```python
from build123d import *

# Parameters (mm, degrees)
F0_R     = 12
F1_DEPTH = 3


with BuildPart() as f1:
    # F0 (on Top) → F1 (new body)
    with BuildSketch(Plane.XY):
        with BuildLine():
            Line((5, 16.248077), (5, 122.001923))
            ThreePointArc((5, 122.001923), (0, 155.25), (-5, 122.001923))
            Line((-5, 122.001923), (-5, 16.248077))
            ThreePointArc((-5, 16.248077), (-8.5, 14.722432), (-11.571247, 12.454165))
            Line((-11.571247, 12.454165), (-103.156765, 65.331089))
            ThreePointArc((-103.156765, 65.331089), (-134.450444, 77.625), (-108.156765, 56.670835))
            Line((-108.156765, 56.670835), (-16.571247, 3.793911))
            ThreePointArc((-16.571247, 3.793911), (-17, 0), (-16.571247, -3.793911))
            Line((-16.571247, -3.793911), (-108.156765, -56.670835))
            ThreePointArc((-108.156765, -56.670835), (-134.450444, -77.625), (-103.156765, -65.331089))
            Line((-103.156765, -65.331089), (-11.571247, -12.454165))
            ThreePointArc((-11.571247, -12.454165), (-8.5, -14.722432), (-5, -16.248077))
            Line((-5, -16.248077), (-5, -122.001923))
            ThreePointArc((-5, -122.001923), (0, -155.25), (5, -122.001923))
            Line((5, -122.001923), (5, -16.248077))
            ThreePointArc((5, -16.248077), (8.5, -14.722432), (11.571247, -12.454165))
            Line((11.571247, -12.454165), (103.156765, -65.331089))
            ThreePointArc((103.156765, -65.331089), (134.450444, -77.625), (108.156765, -56.670835))
            Line((108.156765, -56.670835), (16.571247, -3.793911))
            ThreePointArc((16.571247, -3.793911), (17, 0), (16.571247, 3.793911))
            Line((16.571247, 3.793911), (108.156765, 56.670835))
            ThreePointArc((108.156765, 56.670835), (134.450444, 77.625), (103.156765, 65.331089))
            Line((103.156765, 65.331089), (11.571247, 12.454165))
            ThreePointArc((11.571247, 12.454165), (8.5, 14.722432), (5, 16.248077))
        make_face()
        with Locations((-119.728012, -69.125)):
            Circle(F0_R, mode=Mode.SUBTRACT)
        with Locations((0, -138.25)):
            Circle(F0_R, mode=Mode.SUBTRACT)
        with Locations((119.728012, -69.125)):
            Circle(F0_R, mode=Mode.SUBTRACT)
        with Locations((-119.728012, 69.125)):
            Circle(F0_R, mode=Mode.SUBTRACT)
        Circle(F0_R, mode=Mode.SUBTRACT)
        with Locations((119.728012, 69.125)):
            Circle(F0_R, mode=Mode.SUBTRACT)
        with Locations((0, 138.25)):
            Circle(F0_R, mode=Mode.SUBTRACT)
    extrude(amount=F1_DEPTH)


solid = f1.part
```
Input: part model. Units: mm. Frame: model coordinates. Coordinates: 2 decimals unless noted, no trailing zeros. Loops run counter-clockwise (first coordinate to the right, second up) from the corner with the lowest first, then second, coordinate; pieces in that order, holes last.
Q1. Section D-D, the plane y = -44. Return the cut outline in (x, z).
Results are:
outline: (-86.21, 0) - (-66.21, 0) - (-66.21, 3) - (-86.21, 3) - close; (-5, 0) - (5, 0) - (5, 3) - (-5, 3) - close; (66.21, 0) - (86.21, 0) - (86.21, 3) - (66.21, 3) - close
Q2. Section B-B, the plane x = 0. Return the cut outline in (y, z), and give its area (4 significant figures).
Results are:
outline: (-155.25, 0) - (-150.25, 0) - (-150.25, 3) - (-155.25, 3) - close; (-126.25, 0) - (-12, 0) - (-12, 3) - (-126.25, 3) - close; (12, 0) - (126.25, 0) - (126.25, 3) - (12, 3) - close; (150.25, 0) - (155.25, 0) - (155.25, 3) - (150.25, 3) - close
area: 715.5 mm2
Q3. Mould query, pull axis Y, two halves, no side actions, for faces 1 (the cylindrical face through (134.101, -78.204, 1.479)), 2 (the flat face through (-0.6, 12.2, 0)), 3 (the flat face through (61.72, 29.86, 1.48)). Classes: +Y half, -Y half, draft (parallel to the pull), parting line (faces both ways), or undercut.
Results are:
face 1: undercut
face 2: draft
face 3: undercut
Q4. Line query: line 1 along X through (y, z) = (-26.5, 2.35); line 2 along X through (y, z) = (-30.5, 1.1); line 3 along X through (y, z) = (66, 2.45). Output: solid intervals per line, ascending.
Results are:
line 1: x = -55.9 to -35.9, -5 to 5, 35.9 to 55.9
line 2: x = -62.83 to -42.83, -5 to 5, 42.83 to 62.83
line 3: x = -136.44 to -131.31, -108.14 to -103.02, -5 to 5, 103.02 to 108.14, 131.31 to 136.44
Q5. Contact query for a flat-ended pin moving along its axis: pin 1 (1 mm diameter, centred on y = 27, z = 1, fed in from +X). Output: stop coordinate, or through.
Results are:
pin 1: stops at x = 57.63
Q6. Section A-A, the plane y = 138.25. Return the cut outline in (x, z).
Results are:
outline: (-17, 0) - (-12, 0) - (-12, 3) - (-17, 3) - close; (12, 0) - (17, 0) - (17, 3) - (12, 3) - close
Q7. Section C-C, the plane z = 2.2. Give the number of separate pieces and of enclosed holes in the cut face, and give its area (3 significant figures).
Results are:
separate pieces: 1
enclosed holes: 7
area: 9,470 mm2
